Source: CAD feature listing. Evaluate the final solid. Frame: model axes, mm. Face numbers are marked on the shaded views. Give positions to 0.01 mm unless a question says otherwise; leave off trailing zeros. Loops run counter-clockwise (first coordinate to the right, second up) from the corner with the lowest first, then second, coordinate; pieces in that order, holes last. Notation, with made-up numbers: (-0.75, 79) -> (37.25, 79) arc R5 ccw to (37.25, 87) -> close; hole circle Ø8 at (87, 81.5). An arc over 180 degrees is marked (long way). Return JSON: item names as keys, results as strings. Group by question number.
(1) Draft query along Y for the marked faces 1, 2 and 3. Return one class per face: released by +Y, released by -Y, zero draft, split by the parting line, or undercut.
(2) Cut plane C-C on y = -14.25. Return loops of the section in (x, z), then the cut area to 3 significant figures.
(3) Cut plane A-A on x = 0.75. Return loops of the section in (y, z), then the cut area to 3 significant figures.
(4) Ray query, line 1 (X direction, y = -4.5, z = 1.15); line 2 (Y direction, x = -13, z = 1.2); line 3 (Y direction, x = -6.25, z = 1.1). Return the intervals inside material, ascending. Write a range as from..to.
(5) Pin query (flat end, axial travel): pin 1 (1.5 mm diameter, centred on x = -9.5, y = -20, fed in from -Z). Return the tip coordinate at first contact, or that it passes through.
(6) Cut plane B-B on x = -6. Return loops of the section in (y, z).
(7) Cut plane D-D on y = -17.75. Return loops of the section in (x, z), then the cut area to 3 significant figures.
```python
from build123d import *

# Parameters (mm, degrees)
CROQUIS1_R              = 5
CROQUIS1_R_2            = 1.1
SALIENTE_EXTRUIR1_DEPTH = 2
CORTAR_EXTRUIR1_START   = -2
CORTAR_EXTRUIR1_DEPTH   = 2


with BuildPart() as part:
    # Croquis1 → Saliente-Extruir1 (new body)
    with BuildSketch(Plane.XY):
        with BuildLine():
            Line((-18.543218985, -0.988325299), (-18.543218985, -21.988325299))
            ThreePointArc((-18.543218985, -21.988325299), (-17.957432547, -23.402538861), (-16.543218985, -23.988325299))
            Line((-16.543218985, -23.988325299), (4.456781015, -23.988325299))
            ThreePointArc((4.456781015, -23.988325299), (5.870994578, -23.402538861), (6.456781015, -21.988325299))
            Line((6.456781015, -21.988325299), (6.456781015, -0.988325299))
            ThreePointArc((6.456781015, -0.988325299), (5.870994578, 0.425888264), (4.456781015, 1.011674701))
            Line((4.456781015, 1.011674701), (-16.543218985, 1.011674701))
            ThreePointArc((-16.543218985, 1.011674701), (-17.957432547, 0.425888264), (-18.543218985, -0.988325299))
        make_face()
        with Locations((-6.043218985, -11.488325299)):
            Circle(CROQUIS1_R, mode=Mode.SUBTRACT)
        with Locations((-13.114286796, -4.417257487)):
            Circle(CROQUIS1_R_2, mode=Mode.SUBTRACT)
        with Locations((1.027848827, -4.417257487)):
            Circle(CROQUIS1_R_2, mode=Mode.SUBTRACT)
        with Locations((-13.114286796, -18.559393111)):
            Circle(CROQUIS1_R_2, mode=Mode.SUBTRACT)
        with Locations((1.027848827, -18.559393111)):
            Circle(CROQUIS1_R_2, mode=Mode.SUBTRACT)
    extrude(amount=SALIENTE_EXTRUIR1_DEPTH)

    # Croquis2 → Cortar-Extruir1 (cut)
    with BuildSketch(Plane.XY.offset(2).offset(CORTAR_EXTRUIR1_START)):
        with BuildLine():
            Line((4.456781015, 1.011674701), (-16.543218985, 1.011674701))
            ThreePointArc((-16.543218985, 1.011674701), (-17.957432547, 0.425888264), (-18.543218985, -0.988325299))
            Line((-18.543218985, -0.988325299), (-18.543218985, -21.988325299))
            ThreePointArc((-18.543218985, -21.988325299), (-17.957432547, -23.402538861), (-16.543218985, -23.988325299))
            Line((-16.543218985, -23.988325299), (4.456781015, -23.988325299))
            ThreePointArc((4.456781015, -23.988325299), (5.870994578, -23.402538861), (6.456781015, -21.988325299))
            Line((6.456781015, -21.988325299), (6.456781015, -0.988325299))
            ThreePointArc((6.456781015, -0.988325299), (5.870994578, 0.425888264), (4.456781015, 1.011674701))
        make_face()
        with BuildLine():
            Line((-18.193218985, -0.988325299), (-18.193218985, -21.988325299))
            ThreePointArc((-18.193218985, -21.988325299), (-17.709945174, -23.155051488), (-16.543218985, -23.638325299))
            Line((-16.543218985, -23.638325299), (4.456781015, -23.638325299))
            ThreePointArc((4.456781015, -23.638325299), (5.623507204, -23.155051488), (6.106781015, -21.988325299))
            Line((6.106781015, -21.988325299), (6.106781015, -0.988325299))
            ThreePointArc((6.106781015, -0.988325299), (5.623507204, 0.17840089), (4.456781015, 0.661674701))
            Line((4.456781015, 0.661674701), (-16.543218985, 0.661674701))
            ThreePointArc((-16.543218985, 0.661674701), (-17.709945174, 0.17840089), (-18.193218985, -0.988325299))
        make_face(mode=Mode.SUBTRACT)
    extrude(amount=CORTAR_EXTRUIR1_DEPTH, mode=Mode.SUBTRACT)


solid = part.part
```
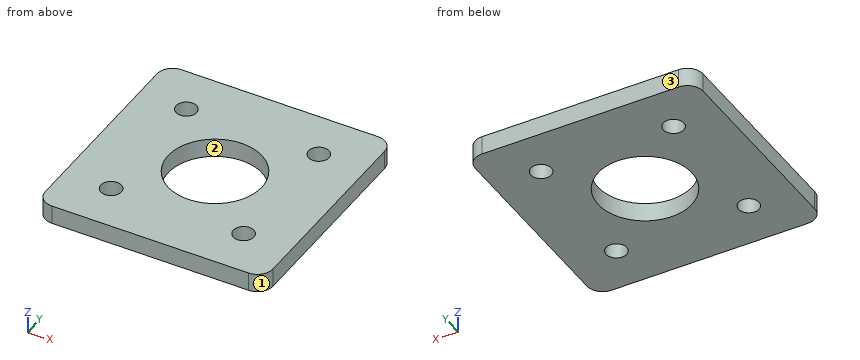
Answers:
{
 "1": {"face 1": "released by -Y", "face 2": "undercut", "face 3": "released by +Y"},
 "2": {"outline": "(-18.19, 0) -> (-10.21, 0) -> (-10.21, 2) -> (-18.19, 2) -> close; (-1.88, 0) -> (6.11, 0) -> (6.11, 2) -> (-1.88, 2) -> close", "area": "31.9 mm²"},
 "3": {"outline": "(-23.64, 0) -> (-19.62, 0) -> (-19.62, 2) -> (-23.64, 2) -> close; (-17.5, 0) -> (-5.48, 0) -> (-5.48, 2) -> (-17.5, 2) -> close; (-3.35, 0) -> (0.66, 0) -> (0.66, 2) -> (-3.35, 2) -> close", "area": "40.1 mm²"},
 "4": {"line 1": "-18.19..-14.21, -12.02..-0.07, 2.12..6.11", "line 2": "-23.64..-19.65, -17.47..-5.51, -3.32..0.66", "line 3": "-23.64..-16.48, -6.49..0.66"},
 "5": {"pin 1": "z = 0"},
 "6": {"outline": "(-23.64, 0) -> (-16.49, 0) -> (-16.49, 2) -> (-23.64, 2) -> close; (-6.49, 0) -> (0.66, 0) -> (0.66, 2) -> (-6.49, 2) -> close"},
 "7": {"outline": "(-18.19, 0) -> (-13.86, 0) -> (-13.86, 2) -> (-18.19, 2) -> close; (-12.37, 0) -> (0.28, 0) -> (0.28, 2) -> (-12.37, 2) -> close; (1.77, 0) -> (6.11, 0) -> (6.11, 2) -> (1.77, 2) -> close", "area": "42.6 mm²"}
}
